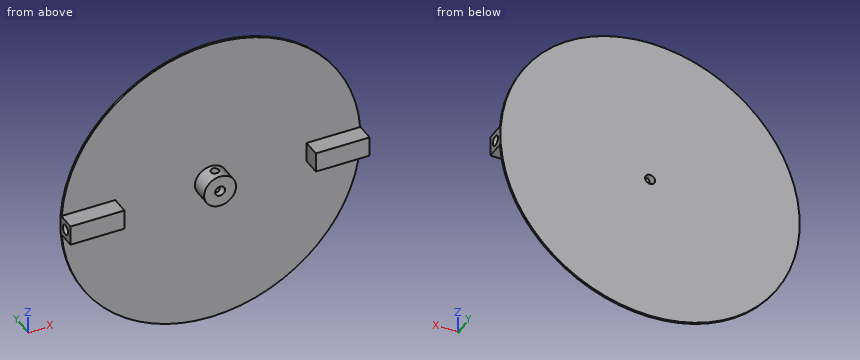
```python
from build123d import *

# Parameters (mm, degrees)
F0_W          = 27
F0_H          = 10
F1_DEPTH      = 10
F0_R          = 2.5
F2_R          = 75
F2_R_2        = 2.5
F3_DEPTH      = 1
F4_R          = 2.5
F5_DEPTH      = 25
F6_R          = 2
F7_DEPTH      = 75.001
F7_DEPTH_BACK = 75.001


# Not quite as in the source:
# - a pattern or mirror of a feature is missing from the dataset's text; its kind, count and spacing are read off the source's solid


with BuildPart() as f1:
    # F0 (on Front) → F1 (new body)
    with BuildSketch(Plane.XZ):
        with Locations((61.5, 0)):
            Rectangle(F0_W, F0_H)
    extrude(amount=F1_DEPTH)



with BuildPart() as f1b:
    # F0 (on Front) → F1, piece 2 (new body)
    with BuildSketch(Plane.XZ):
        with Locations((-61.5, 0)):
            Rectangle(F0_W, F0_H)
    extrude(amount=F1_DEPTH)


with BuildPart() as f1c:
    # F0 (on Front) → F1, piece 3 (new body)
    with BuildSketch(Plane.XZ):
        with BuildLine():
            ThreePointArc((6.2449979984, 5), (0, 8), (-6.2449979984, 5))
            ThreePointArc((-6.2449979984, 5), (-8, 0), (-6.2449979984, -5))
            ThreePointArc((-6.2449979984, -5), (0, -8), (6.2449979984, -5))
            ThreePointArc((6.2449979984, -5), (8, 0), (6.2449979984, 5))
        make_face()
        Circle(F0_R, mode=Mode.SUBTRACT)
    extrude(amount=F1_DEPTH)


with BuildPart() as f1_1:
    add(f1.part)

    add(f1b.part)  # F3 merges F1b

    add(f1c.part)  # F3 merges F1c
    # F2 (on face) → F3 (join)
    with BuildSketch(Plane(origin=(0, 0, 0), x_dir=(-1, 0, 0), z_dir=(0, 1, 0))):
        Circle(F2_R)
        Circle(F2_R_2, mode=Mode.SUBTRACT)
    extrude(amount=-F3_DEPTH)

    # F4 (on face) → F5 (cut)
    with BuildSketch(Plane(origin=(-75, 0, 0), x_dir=(0, -1, 0), z_dir=(-1, 0, 0))):
        with Locations((5, 0)):
            Circle(F4_R)
    f5 = extrude(amount=-F5_DEPTH, mode=Mode.SUBTRACT)

    # F5_copies: F5 across plane
    add(f5.mirror(Plane(origin=(0, 0, 0), x_dir=(0, 0, 1), z_dir=(1, 0, 0))), mode=Mode.SUBTRACT)

    # F6 (on Top) → F7 (cut, two sides)
    with BuildSketch(Plane.XY) as f7_sk:
        with Locations((0, -5)):
            Circle(F6_R)
    extrude(amount=-F7_DEPTH, mode=Mode.SUBTRACT)
    extrude(f7_sk.sketch, amount=F7_DEPTH_BACK, mode=Mode.SUBTRACT)


solid = f1_1.part
```
Geometry check sheet. Reference: the model listing, model coordinates, mm. Round coordinates to 2 decimals unless told otherwise and drop trailing zeros. Write each loop counter-clockwise with the first axis right and the second up, starting at its lowest first coordinate (ties: lowest second). Pieces come first, ordered by that corner, then holes. Notation, with made-up numbers: (82.5, 85.5) -> (130.5, 85.5) arc R20 ccw to (130.5, 108.5) -> close; hole circle Ø1 at (17.25, 70). An arc over 180 degrees is marked (long way). Put each result on its own line as item: value.
1) Cross-section at C-C, the plane y = -5. Enter the section's corners in (x, z), plus the area to 3 significant figures.
Recorded:
outline: (-75, -5) -> (-48, -5) -> (-48, 5) -> (-75, 5) -> (-75, 2.5) -> (-50, 2.5) -> (-50, -2.5) -> (-75, -2.5) -> close; (-2, -7.75) -> (-2, -1.5) arc R2.5 cw to (-2, 1.5) -> (-2, 7.75) arc R8 ccw to start; (2, -7.75) arc R8 ccw to (2, 7.75) -> (2, 1.5) arc R2.5 cw to (2, -1.5) -> close; (48, -5) -> (75, -5) -> (75, -2.5) -> (50, -2.5) -> (50, 2.5) -> (75, 2.5) -> (75, 5) -> (48, 5) -> close
area: 426 mm2
2) Cross-section at B-B, the plane x = 58.5. Enter the section's corners in (y, z), plus the area to 3 significant figures.
Recorded:
outline: (-10, -5) -> (-1, -5) -> (-1, -46.93) -> (0, -46.93) -> (0, 46.93) -> (-1, 46.93) -> (-1, 5) -> (-10, 5) -> close; hole circle Ø5 at (-5, 0)
area: 164 mm2
3) Cross-section at D-D, the plane z = -37.5. Enter the section's corners in (x, y), plus the area to 3 significant figures.
Recorded:
outline: (-64.95, -1) -> (64.95, -1) -> (64.95, 0) -> (-64.95, 0) -> close
area: 130 mm2
4) Thickness scan on probe 1 along Y at (x, z) = (0, 5); probe 2 along Y at (x, z) = (-26, -15); probe 3 along Z at (x, y) = (2, -0.75). Record the ranges inside material, lowest first. Write a range as from..to.
Recorded:
probe 1: y = -10..-7, -3..0
probe 2: y = -1..0
probe 3: z = -74.97..-1.5, 1.5..74.97
5) Cross-section at A-A, the plane x = 0. Enter the section's corners in (y, z), plus the area to 3 significant figures.
Recorded:
outline: (-10, -8) -> (-7, -8) -> (-7, -2.5) -> (-10, -2.5) -> close; (-10, 2.5) -> (-7, 2.5) -> (-7, 8) -> (-10, 8) -> close; (-3, -8) -> (-1, -8) -> (-1, -75) -> (0, -75) -> (0, -2.5) -> (-3, -2.5) -> close; (-3, 2.5) -> (0, 2.5) -> (0, 75) -> (-1, 75) -> (-1, 8) -> (-3, 8) -> close
area: 200 mm2
6) Depth check by flat-ended pin: P1, Ø3, axis at x = 0, y = -5, coming from the -Z side; P2, Ø3, axis at x = -58.5, y = -1, coming from the +Z side; P3, Ø3, axis at x = -43, z = 16.5, coming from the -Y side; P4, Ø3, axis at y = -5, z = 0, coming from the -X side. Enter the tip coordinate at first touch or a pass-through.
Recorded:
P1: passes through
P2: stops at z = 48.74
P3: stops at y = -1
P4: stops at x = -50
